from build123d import *

# Parameters (mm, degrees)
F1_DEPTH = 4.7625


# Not quite as in the source:
# - a feature of the source that left no trace in its solid (it failed there, or was rolled back) is left out


with BuildPart() as f1:
    # F0 (on Top) → F1 (new body)
    with BuildSketch(Plane.XY):
        with BuildLine():
            Line((-6.7869197201, 18.6999163445), (-29.9817704813, 31.019788517))
            Line((-29.9817704813, 31.019788517), (-18.4581812066, 7.4192113543))
            ThreePointArc((-18.4581812066, 7.4192113543), (-11.2260431578, 1.9743769297), (-19.8819508265, -0.6761522815))
            Line((-19.8819508265, -0.6761522815), (-38.7664486034, -18.9287163727))
            Line((-38.7664486034, -18.9287163727), (-12.7599809824, -15.2621111222))
            ThreePointArc((-12.7599809824, -15.2621111222), (-5.3467821599, -10.0664854729), (-5.5008016534, -19.117801436))
            Line((-5.5008016534, -19.117801436), (6.0227876213, -42.7183785987))
            Line((6.0227876213, -42.7183785987), (10.5720792637, -16.8517147679))
            ThreePointArc((10.5720792637, -16.8517147679), (7.9215500525, -8.1958070991), (16.4822684394, -11.1392987961))
            Line((16.4822684394, -11.1392987961), (42.4887360604, -7.4726935456))
            Line((42.4887360604, -7.4726935456), (19.2938852991, 4.8471786269))
            ThreePointArc((19.2938852991, 4.8471786269), (10.242569336, 5.0011981203), (15.6874037606, 12.2333361692))
            Line((15.6874037606, 12.2333361692), (20.236695403, 38.1))
            Line((20.236695403, 38.1), (1.3521976262, 19.8474359089))
            ThreePointArc((1.3521976262, 19.8474359089), (-1.5912940708, 11.286717522), (-6.7869197201, 18.6999163445))
        make_face()
    extrude(amount=F1_DEPTH)


solid = f1.part
Read the model definition and answer for the solid it produces. Units are mm, in the model's axes. A direction names the side the tool comes from. Give positions to 0.01 mm unless a question says otherwise; leave off trailing zeros. Write each loop counter-clockwise with the first axis right and the second up, starting at its lowest first coordinate (ties: lowest second). Pieces come first, ordered by that corner, then holes. Notation, with made-up numbers: (8.5, 45) -> (33.5, 45) arc R29 ccw to (33.5, 72) -> close; hole circle Ø7 at (-18.75, -29.75). An arc over 180 degrees is marked (long way). Answer as a JSON object with one key per item and string values. Group by question number.
1) Find section B-B (y = 23). Write down the section's boundary in (x, z).
2) Find section C-C (z = 0.85). Write down the section's boundary in (x, y), and give its area (3 significant figures).
3) Find section D-D (y = -34.5). Write down the section's boundary in (x, z), and give its area (3 significant figures).
4) The mould has two halves that part along X. Classify faces 1 (the flat face through (29.303, -9.332, 2.348)), 2 (the flat face through (-25.95, -17.12, 2.35)), 3 (the flat face through (0.18, -30.75, 2.35)): +X half, -X half, draft (parallel to the pull), parting line (faces both ways), or undercut.
5) Consider L1, parallel to Y at x = -4, z = 3.8; L2, parallel to X at y = 16, z = 2.3; L3, parallel to Y at x = 11.5, z = 2.7. Determine where each line is inside the solid, lowest interval first. Write a range as from..to.
6) This flat-tipped pin is pushed along its axis until it touches: P1, Ø1.5, axis at x = 9.5, z = 3, coming from the +Y side. Where does it stop, or does it pass through?
7) A tool of negligible diameter and unlimited length cuts with its end or side. For faces 4 (the flat face through (2, -2, 4.762)), 5 (the flat face through (-24.3, 19.38, 2.35)), 6 (the flat face through (10.927, 29.101, 2.348)), 7 (the flat face through (17.93, 24.99, 2.35)), from which of +Z, -Z, +X, -X, +Y, -Y can it reach the whole face along a straight path? Write none if from no direction.
8) Find section A-A (x = -4). Write down the section's boundary in (y, z).
Values follow:
{
 "1": {"outline": "(-26.07, 0) -> (-14.88, 0) -> (-14.88, 4.76) -> (-26.07, 4.76) -> close; (4.61, 0) -> (17.58, 0) -> (17.58, 4.76) -> (4.61, 4.76) -> close"},
 "2": {"outline": "(-38.77, -18.93) -> (-12.76, -15.26) arc R5.08 cw (long way) to (-5.5, -19.12) -> (6.02, -42.72) -> (10.57, -16.85) arc R5.08 cw (long way) to (16.48, -11.14) -> (42.49, -7.47) -> (19.29, 4.85) arc R5.08 cw (long way) to (15.69, 12.23) -> (20.24, 38.1) -> (1.35, 19.85) arc R5.08 cw (long way) to (-6.79, 18.7) -> (-29.98, 31.02) -> (-18.46, 7.42) arc R5.08 cw (long way) to (-19.88, -0.68) -> close", "area": "1,810 mm2"},
 "3": {"outline": "(2.01, 0) -> (7.47, 0) -> (7.47, 4.76) -> (2.01, 4.76) -> close", "area": "26.0 mm2"},
 "4": {"face 1": "+X half", "face 2": "undercut", "face 3": "-X half"},
 "5": {"L1": "y = -22.19..-18, -11.1..11.53", "L2": "x = -22.65..-7.37, 2.77..16.35", "L3": "y = -6.77..3.37, 11.09..29.66"},
 "6": {"P1": "stops at y = 28.45"},
 "7": {"face 4": "+Z, +X, -X, +Y, -Y", "face 5": "+Z, -Z, -X", "face 6": "+Z, -Z, +Y", "face 7": "+Z, -Z, +X"},
 "8": {"outline": "(-22.19, 0) -> (-18, 0) -> (-18, 4.76) -> (-22.19, 4.76) -> close; (-11.1, 0) -> (11.53, 0) -> (11.53, 4.76) -> (-11.1, 4.76) -> close"}
}
